Autodesk Inventor part; units mm, degrees
ref_plane "Work Plane1" through (0, 0, 10.5) normal (1, 0, 0) x (0, 0, -1)
ref_plane "YZ Plane" through (0, 0, 0) normal (1, 0, 0) x (0, 1, 0)
ref_plane "XZ Plane" through (0, 0, 0) normal (0, 1, 0) x (-1, 0, 0)
sketch "Sketch1" plane through (0, 0, 0) normal (0, 1, 0) x (-1, 0, 0)
  line L0 (-15, 21) -> (15, 21)
  line L1 (15, 21) -> (15, -21)
  line L2 (15, -21) -> (-15, -21)
  line L3 (-15, -21) -> (-15, 21)
  line L4 (-15, 21) -> (15, -21) construction
  line L5 (15, 21) -> (-15, -21) construction
  line L6 (-9.525, 16.6751) -> (9.525, 16.6751) construction
  line L7 (9.525, 16.6751) -> (9.525, -16.6751) construction
  line L8 (9.525, -16.6751) -> (-9.525, -16.6751) construction
  line L9 (-9.525, -16.6751) -> (-9.525, 16.6751) construction
  line L10 (-9.525, 16.6751) -> (9.525, -16.6751) construction
  line L11 (9.525, 16.6751) -> (-9.525, -16.6751) construction
  circle A0 centre (9.525, 16.6751) radius 2.032
  circle A1 centre (-9.525, -16.6751) radius 2.032
  circle A2 centre (9.525, -16.6751) radius 2.032
  circle A3 centre (-9.525, 16.6751) radius 2.032
  point P0 (0, 0)
  dimension "d0" = 30
  dimension "d1" = 42
  dimension "d2" = 33.3502
  dimension "d3" = 19.05
  dimension "d6" = 4.064
  dimension "d7" = 4.064
  dimension "d36" = 4.064
  dimension "d37" = 4.064
extrude "Extrusion1" add sketch "Sketch1" against normal blind 3
sketch "Sketch2" plane through (0, 0, 0) normal (0, 1, 0) x (1, 0, 0)
  line L0 (27.5, -12.5) -> (-27.5, -12.5)
  line L1 (-27.5, -12.5) -> (-27.5, 12.5)
  line L2 (-27.5, 12.5) -> (27.5, 12.5)
  line L3 (27.5, 12.5) -> (27.5, -12.5)
  line L4 (27.5, -12.5) -> (-27.5, 12.5) construction
  line L5 (-27.5, -12.5) -> (27.5, 12.5) construction
  point P0 (0, 0)
  point P1 (0, 0)
  point P2 (0, 0)
  dimension "d9" = 25
  dimension "d13" = 55
extrude "Extrusion2" add sketch "Sketch2" along normal blind 19
sketch "Sketch3" plane through (27.5, 0, 12.5) normal (1, 0, 0) x (0, 0, -1)
  line L0 (25, 0) -> (0, 0)
  line L1 (25, 0) -> (25, 19)
  line L2 (0, 19) -> (25, 19)
  line L3 (0, 0) -> (0, 19)
  line L4 (33.5, 0) -> (25, 0)
  line L5 (25, 0) -> (0, 0)
  line L6 (0, 0) -> (-8.5, 0)
  line L7 (-8.5, 0) -> (-8.5, -3)
  line L8 (33.5, -3) -> (-8.5, -3)
  line L9 (33.5, 0) -> (33.5, -3)
  circle A0 centre (12.5, 8) radius 7.7
  point P0 (12.5, 0)
  point P1 (12.5, 0)
  point P2 (12.5, 0)
  dimension "d12" = 15.4
  dimension "d28" = 11
extrude "Extrusion3" cut sketch "Sketch3" against normal through all contours A0
fillet "Fillet1" radius 10 2 edges at (0, 19, -12.5) (0, 19, 12.5)
fillet "Fillet2" radius 2 10 edges at (27.5, 19, 0) (27.5, 16.0711, -9.5711) (27.5, 4.5, -12.5) (27.5, 4.5, 12.5) (27.5, 16.0711, 9.5711) (-27.5, 19, 0) (-27.5, 16.0711, 9.5711) (-27.5, 4.5, 12.5) (-27.5, 4.5, -12.5) (-27.5, 16.0711, -9.5711)
fillet "Fillet3" radius 1 2 edges at (0, 0, 21) (0, 0, -21)
sketch "Sketch4" plane through (0, 19, 0) normal (0, 1, 0) x (1, 0, 0)
  line L0 (26.2, -8.1) -> (24.1, -8.1)
  line L1 (24.1, -8.1) -> (24.1, 8.1)
  line L2 (24.1, 8.1) -> (26.2, 8.1)
  line L3 (26.2, 8.1) -> (26.2, -8.1)
  line L4 (25.5, -2.5) -> (-25.5, -2.5)
  line L5 (-25.5, 2.5) -> (25.5, 2.5)
  line L6 (-25.5, -2.5) -> (-25.5, 2.5)
  line L7 (25.5, 2.5) -> (25.5, -2.5)
  point P0 (0, 0)
  dimension "d16" = 24.1
  dimension "d18" = 2.1
  dimension "d34" = 8.1
  dimension "d35" = 8.1
extrude "Extrusion4" cut sketch "Sketch4" against normal blind 6.1 contours L0 L1 L4 L7 L5 L2 L3 | L1 L5 L7 L4
ref_plane "Work Plane1" through (0, 0, 10.5) normal (1, 0, 0) x (0, 0, -1)
mirror "Mirror1" about plane through (0, 0, 10.5) normal (1, 0, 0) of "Extrusion4"
sketch "Sketch5" plane through (0, 12.9, 0) normal (0, 1, 0) x (1, 0, 0)
  line L0 (26.2, 9.4632) -> (26.2, -9.4632)
  line L1 (24.1, -9.6414) -> (24.1, 9.6414)
  line L2 (-24.1, 9.6414) -> (-24.1, -9.6414)
  line L3 (-26.2, -9.4632) -> (-26.2, 9.4632)
  line L4 (26.2, -9.5) -> (24.1, -9.5)
  line L5 (24.1, -9.5) -> (24.1, 9.5)
  line L6 (24.1, 9.5) -> (26.2, 9.5)
  line L7 (26.2, 9.5) -> (26.2, -9.5)
  line L8 (-24.1, -9.5) -> (-26.2, -9.5)
  line L9 (-26.2, -9.5) -> (-26.2, 9.5)
  line L10 (-26.2, 9.5) -> (-24.1, 9.5)
  line L11 (-24.1, 9.5) -> (-24.1, -9.5)
  line L12 (-25.5, 9.6414) -> (-24.1, 9.6414)
  line L13 (-24.1, -9.6414) -> (-25.5, -9.6414)
  line L14 (-25.5, 9.6414) -> (-24.1, 9.6414)
  line L15 (-24.1, -9.6414) -> (-25.5, -9.6414)
  line L16 (24.1, 9.6414) -> (25.5, 9.6414)
  line L17 (24.1, -9.6414) -> (24.1, 9.6414)
  line L18 (25.5, -9.6414) -> (24.1, -9.6414)
  line L19 (26.2, 9.4632) -> (26.2, -9.4632)
  line L20 (24.1, 9.6414) -> (25.5, 9.6414)
  line L21 (25.5, -9.6414) -> (24.1, -9.6414)
  line L22 (-24.1, 9.6414) -> (-24.1, -9.6414)
  line L23 (-26.2, -9.4632) -> (-26.2, 9.4632)
  point P0 (0, 0)
properties part number "slave-slider-house"
Check sheet for the modelled part. Datum: model origin and axes. Units: mm. A direction names the side the tool comes from. Coordinates: 2 decimals unless noted, no trailing zeros. Loops run counter-clockwise (first coordinate to the right, second up) from the corner with the lowest first, then second, coordinate; pieces in that order, holes last. Notation, with made-up numbers: M 38,12.25 L 86,12.25 A32 ccw 86,39.25 Z; hole C 80.25,41 d11. An arc over 180 degrees is marked long. Answer as a JSON object with one key per item and string values.
1. Sectioned sample at D-D on x = -1.5. Record the cut outline in (y, z).
Outcome:
{"outline": "M -3,-21 L -1,-21 A1 ccw 0,-20 L 0,-12.5 L 9,-12.5 A10 ccw 19,-2.5 L 19,2.5 A10 ccw 9,12.5 L 0,12.5 L 0,20 A1 ccw -1,21 L -3,21 Z; hole C 8,0 d15.4"}
2. Scan lines: L1, parallel to Y at x = -1, z = 0; L2, parallel to Z at x = 8, y = -0.75; L3, parallel to Y at x = 4.5, z = 16.5. Record each from-to range of solid material in increasing order. Write a range as from..to.
Outcome:
{"L1": "-3..0.3, 15.7..19", "L2": "-20.97..-18.02, -15.33..15.33, 18.02..20.97", "L3": "-3..0"}
3. Release check for a two-part mould opening along Z. For faces 1 (the cylindrical face through (0.36, 15.99, -9.65)), 2 (the flat face through (25, 12.9, -7)), 3 (the flat face through (15, -1, 0)) record: pulls with the +Z half, pulls with the -Z half, needs draft (parallel to the pull), parting line crosses it, or undercut.
Outcome:
{"face 1": "pulls with the -Z half", "face 2": "undercut", "face 3": "needs draft"}
4. Sectioned sample at A-A on y = 8. Record the cut outline in (x, z), and give its area (3 significant figures).
Outcome:
{"outline": "M -27.5,-10.5 A2 ccw -25.5,-12.5 L 25.5,-12.5 A2 ccw 27.5,-10.5 L 27.5,-7.7 L -27.5,-7.7 Z; M -27.5,7.7 L 27.5,7.7 L 27.5,10.5 A2 ccw 25.5,12.5 L -25.5,12.5 A2 ccw -27.5,10.5 Z", "area": "525 mm²"}
5. Depth check by flat-ended pin: P1, Ø1.7, axis at x = -25, z = -6.5, coming from the +Y side; P2, Ø6.5, axis at x = -9.52, z = -16.68, coming from the +Y side; P3, Ø0.6, axis at x = 25.5, y = 14.5, coming from the +Z side; P4, Ø10, axis at x = -11, y = 2.5, coming from the -Z side. Enter the tip coordinate at first touch or a pass-through.
Outcome:
{"P1": "y = 12.9", "P2": "y = 0", "P3": "z = 11.04", "P4": "z = -21"}
6. Sectioned sample at B-B on z = 0. Record the cut outline in (x, y), and give its area (3 significant figures).
Outcome:
{"outline": "M -27.5,0 L -15,0 L -15,-3 L 15,-3 L 15,0 L 27.5,0 L 27.5,0.3 L -27.5,0.3 Z; M -27.5,15.7 L -26.2,15.7 L -26.2,18.87 A2 ccw -27.5,17 Z; M -24.1,15.7 L 24.1,15.7 L 24.1,19 L -24.1,19 Z; M 26.2,15.7 L 27.5,15.7 L 27.5,17 A2 ccw 26.2,18.87 Z", "area": "272 mm²"}
7. Sectioned sample at C-C on x = -21.5. Record the cut outline in (y, z), and give its area (3 significant figures).
Outcome:
{"outline": "M 0,-12.5 L 9,-12.5 A10 ccw 19,-2.5 L 19,2.5 A10 ccw 9,12.5 L 0,12.5 Z; hole C 8,0 d15.4", "area": "246 mm²"}
8. Access from +Z, -Z, +X, -X, +Y, -Y to the whole of each face (thin tool, end or side, straight path). Record for faces 4 (the flat face through (-15, -1, 0)), 5 (the flat face through (27.5, 4.6, -7.1)), 6 (the flat face through (25, 15, -8.1)).
Outcome:
{"face 4": "+Z, -Z, -X, -Y", "face 5": "+Z, -Z, +X, +Y, -Y", "face 6": "+Y"}
